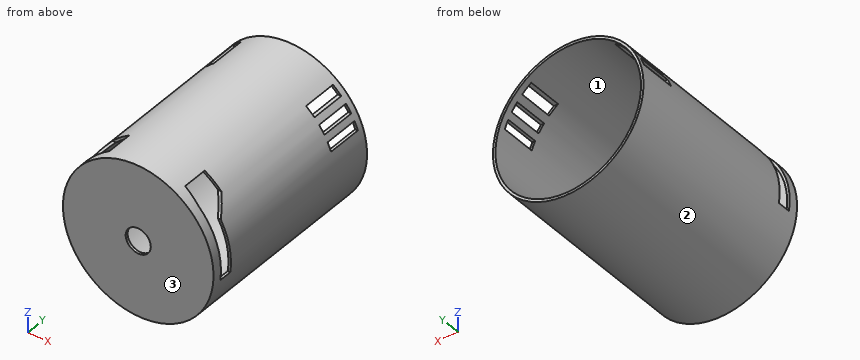
```python
from build123d import *

# Parameters (mm, degrees)
F0_R     = 76.2
F1_DEPTH = 203.2
F2_R     = 12.7
F3_DEPTH = 38.1
F4_T     = -2.54
F5_W     = 35.56
F5_H     = 7.62
F5_H_2   = 8.059159
F6_DEPTH = 88.9
F7_R     = 12.7
F8_DEPTH = 241.301


with BuildPart() as f1:
    # F0 (on Front) → F1 (new body)
    with BuildSketch(Plane.XZ):
        Circle(F0_R)
    extrude(amount=F1_DEPTH)

    # F2 (on face) → F3 (join)
    with BuildSketch(Plane.XZ.offset(203.2)):
        Circle(F2_R)
    extrude(amount=F3_DEPTH)

    # F4
    f4_openings = [f1.faces().sort_by_distance(p)[0] for p in [
        (0, 0, 0),
    ]]
    offset(amount=F4_T, openings=f4_openings)

    # F5 (on Right) → F6 (cut, symmetric)
    with BuildSketch(Plane.YZ):
        with Locations((-24.242766, 56.482356)):
            Rectangle(F5_W, F5_H)
        with Locations((-24.242766, 43.461889)):
            Rectangle(F5_W, F5_H)
        with Locations((-24.242766, 29.646189)):
            Rectangle(F5_W, F5_H_2)
        Polygon((-165.21275, 65.912403), (-191.117182, 65.912403), (-193.419799, 54.399319), (-193.419799, -10.649604), (-180.17976, -10.649604), (-180.17976, 38.281005), (-165.21275, 52.672356), align=None)
    extrude(amount=F6_DEPTH, both=True, mode=Mode.SUBTRACT)

    # F7 (on face) → F8 (cut, through all)
    with BuildSketch(Plane.XZ.offset(241.3)):
        Circle(F7_R)
    extrude(amount=-F8_DEPTH, mode=Mode.SUBTRACT)


solid = f1.part
```
CAD build for the part. Positions are in the model's coordinates, mm. Face numbers are marked on the shaded views. Round coordinates to 2 decimals unless told otherwise and drop trailing zeros. Loops run counter-clockwise (first coordinate to the right, second up) from the corner with the lowest first, then second, coordinate; pieces in that order, holes last. Notation, with made-up numbers: M 87.25,-9.5 L 123.25,-9.5 A26 ccw 123.25,14.5 Z; hole C -38.75,25 d4. An arc over 180 degrees is marked long. Return JSON: item names as keys, results as strings. Group by question number.
(1) Wall check: probe 1 along Z at (x, y) = (0, -159); probe 2 along X at (y, z) = (-68, 10.5). Give the ranges that are in metal, low to high. Write a range as [from, to].
(2) Saw through at A-A, the plane z = 0. List the corners of the cut face in (x, y), and give its area (3 significant figures).
(3) Drop flat-ended pins along their axis: P1, Ø3, axis at x = 21.5, y = -95, coming from the +Z side; P2, Ø8, axis at y = -51.5, z = -48.5, coming from the +X side; P3, Ø1.3, axis at x = 74.5, y = -190, coming from the +Z side; P4, Ø4, axis at x = -62, z = 45, coming from the -Y side. Give the stop position or say it passes through.
(4) Saw through at C-C, the plane y = -66. List the corners of the cut face in (x, z), and give its area (3 significant figures).
(5) Mould opens along X. For the marked faces 1, 2 and 3 say: +X half, -X half, draft (parallel to the pull), parting line (faces both ways), or undercut.
(6) Saw through at B-B, the plane x = 0. List the corners of the cut face in (y, z), and give its area (3 significant figures).
(7) Saw through at D-D, the plane z = -26.5. List the corners of the cut face in (x, y), and give its area (3 significant figures).
Answer list:
{
 "1": {"probe 1": "[-76.2, -73.66], [73.66, 76.2]", "probe 2": "[-75.47, -72.91], [72.91, 75.47]"},
 "2": {"outline": "M -76.2,-203.2 L -12.7,-203.2 L -12.7,-200.66 L -73.66,-200.66 L -73.66,-193.42 L -76.2,-193.42 Z; M -76.2,-180.18 L -73.66,-180.18 L -73.66,0 L -76.2,0 Z; M 12.7,-203.2 L 76.2,-203.2 L 76.2,-193.42 L 73.66,-193.42 L 73.66,-200.66 L 12.7,-200.66 Z; M 73.66,-180.18 L 76.2,-180.18 L 76.2,0 L 73.66,0 Z", "area": "1,270 mm2"},
 "3": {"P1": "z = 73.53", "P2": "x = 61.86", "P3": "z = -10.65", "P4": "y = -203.2"},
 "4": {"outline": "C 0,0 d152.4; hole C 0,0 d147.32", "area": "1,200 mm2"},
 "5": {"face 1": "undercut", "face 2": "parting line", "face 3": "draft"},
 "6": {"outline": "M -203.2,-76.2 L 0,-76.2 L 0,-73.66 L -200.66,-73.66 L -200.66,-12.7 L -203.2,-12.7 Z; M -203.2,12.7 L -200.66,12.7 L -200.66,73.66 L 0,73.66 L 0,76.2 L -203.2,76.2 Z", "area": "1,340 mm2"},
 "7": {"outline": "M -71.44,-203.2 L 71.44,-203.2 L 71.44,0 L 68.73,0 L 68.73,-200.66 L -68.73,-200.66 L -68.73,0 L -71.44,0 Z", "area": "1,450 mm2"}
}
